The figure shows three views and two pictorial views of one solid part (mm, origin at its lowest corner). Answer the questions. Coordinates: 2 decimals unless noted, no trailing zeros. Loops run counter-clockwise (first coordinate to the right, second up) from the corner with the lowest first, then second, coordinate; pieces in that order, holes last.
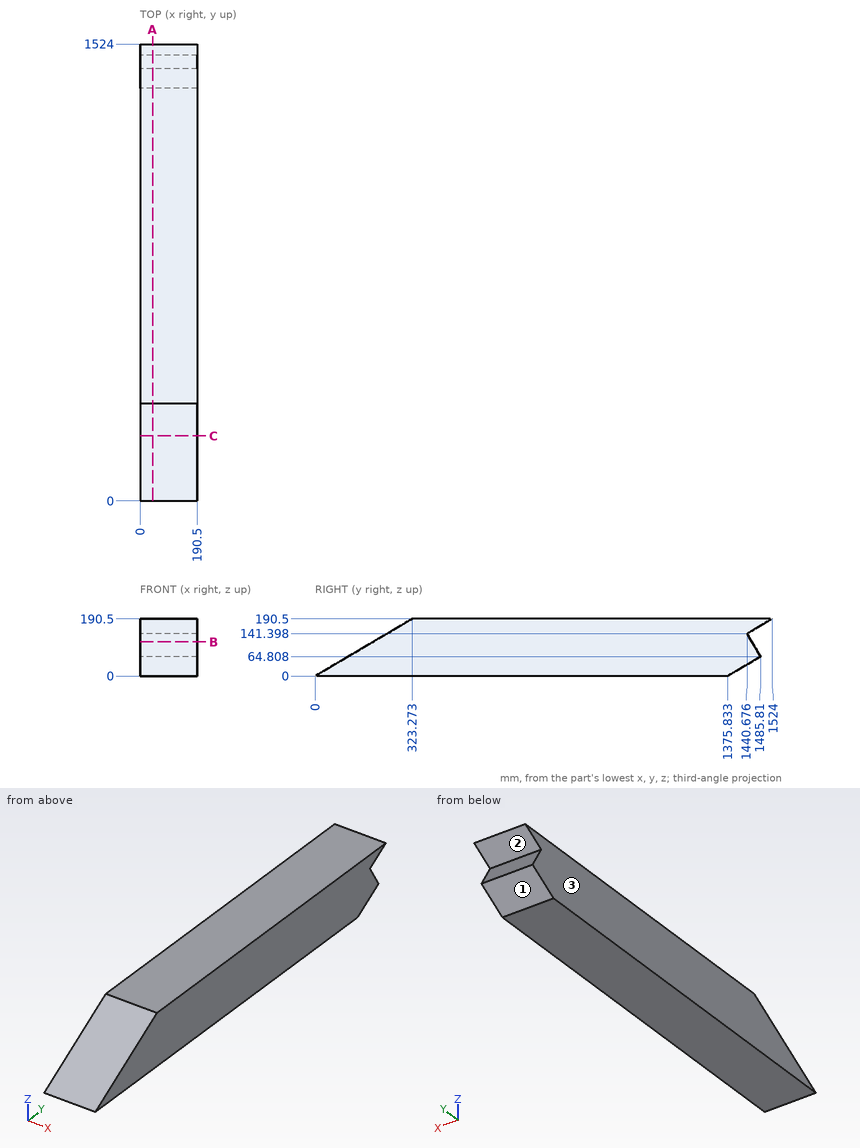
Q1. A cutting plane is placed at C-C (y = 217). Give the vertices of the cut face in (x, z) (1 decimal), then the cut area to 3 significant figures.
Findings below:
outline: (0, 0) - (190.5, 0) - (190.5, 127.9) - (0, 127.9) - close
area: 24,400 mm2
Q2. Flat-ended cylindrical pins translate along their axes: pin 1 Ø5 at (x, z) = (157.5, 96) entering from +Y; pin 2 Ø8 at (x, z) = (159, 53) entering from -Y; pin 3 Ø5 at (x, z) = (90.5, 99.5) entering from +Y. Find the tip coordinate at first contact, or state that the pin passes through.
Findings below:
pin 1: stops at y = 1468.9
pin 2: stops at y = 83.15
pin 3: stops at y = 1466.84
Q3. Determine the mould class of the marked faces 1, 2 and 3 for opening direction Z: +Z half, -Z half, draft (parallel to the pull), parting line (faces both ways), or undercut.
Findings below:
face 1: -Z half
face 2: undercut
face 3: draft
Q4. A cutting plane is placed at A-A (x = 42.5). Give the vertices of the cut face in (y, z), then the cut area to 3 significant figures.
Findings below:
outline: (0, 0) - (1375.83, 0) - (1485.81, 64.81) - (1440.68, 141.4) - (1524, 190.5) - (323.27, 190.5) - close
area: 247,000 mm2
Q5. Straight lines are drawn through the part: probe 1 along Y at (x, z) = (95, 28.5) (1 decimal); probe 2 along Y at (x, z) = (165.5, 139); probe 3 along Z at (x, y) = (121.5, 202) (1 decimal). For each, find the intervals that lie inside material, in ascending order.
Findings below:
probe 1: y = 48.4 to 1424.2
probe 2: y = 235.88 to 1442.09
probe 3: z = 0 to 119
Q6. A cutting plane is placed at B-B (z = 113.5). Give the vertices of the cut face in (x, y).
Findings below:
outline: (0, 192.61) - (190.5, 192.61) - (190.5, 1457.12) - (0, 1457.12) - close
